Check sheet for the drawn part. Datum: minimum x, y, z corner. Units: mm. Coordinates: 2 decimals unless noted, no trailing zeros. Write each loop counter-clockwise with the first axis right and the second up, starting at its lowest first coordinate (ties: lowest second). Pieces come first, ordered by that corner, then holes. Notation, with made-up numbers: M 46.5,64.5 L 57.5,64.5 A28 cw 57.5,96.5 Z; hole C 55,-40 d4. An arc over 180 degrees is marked long. Answer as CSV lines item,"result". Start each with the question number.
Q1. Sectioned sample at B-B, the plane z = 61.13. Record the cut outline in (x, y), then the cut area to 3 significant figures.
Q2. Sectioned sample at D-D, the plane z = 93. Record the cut outline in (x, y).
Q3. Sectioned sample at A-A, the plane y = 1.45. Record the cut outline in (x, z), then the cut area to 3 significant figures.
Q4. Thickness scan on line 1 along Z through (x, y) = (40, 2.2); line 2 along Z through (x, y) = (38, 2.55); line 3 along X through (y, z) = (2.85, 58). Record the ranges inside material, lowest first. Write a range as from..to.
Q5. Sectioned sample at C-C, the plane x = 40. Record the cut outline in (y, z).
Q6. Depth check by flat-ended pin: pin 1 Ø0.9 at (x, y) = (75.5, 1.5) entering from -Z; pin 2 Ø0.9 at (y, z) = (1, 74.5) entering from +X; pin 3 Ø1.5 at (y, z) = (2, 31.5) entering from +X; pin 4 Ø1 at (x, y) = (27.5, 0.5) entering from -Z. Enter the tip coordinate at first touch or a pass-through.
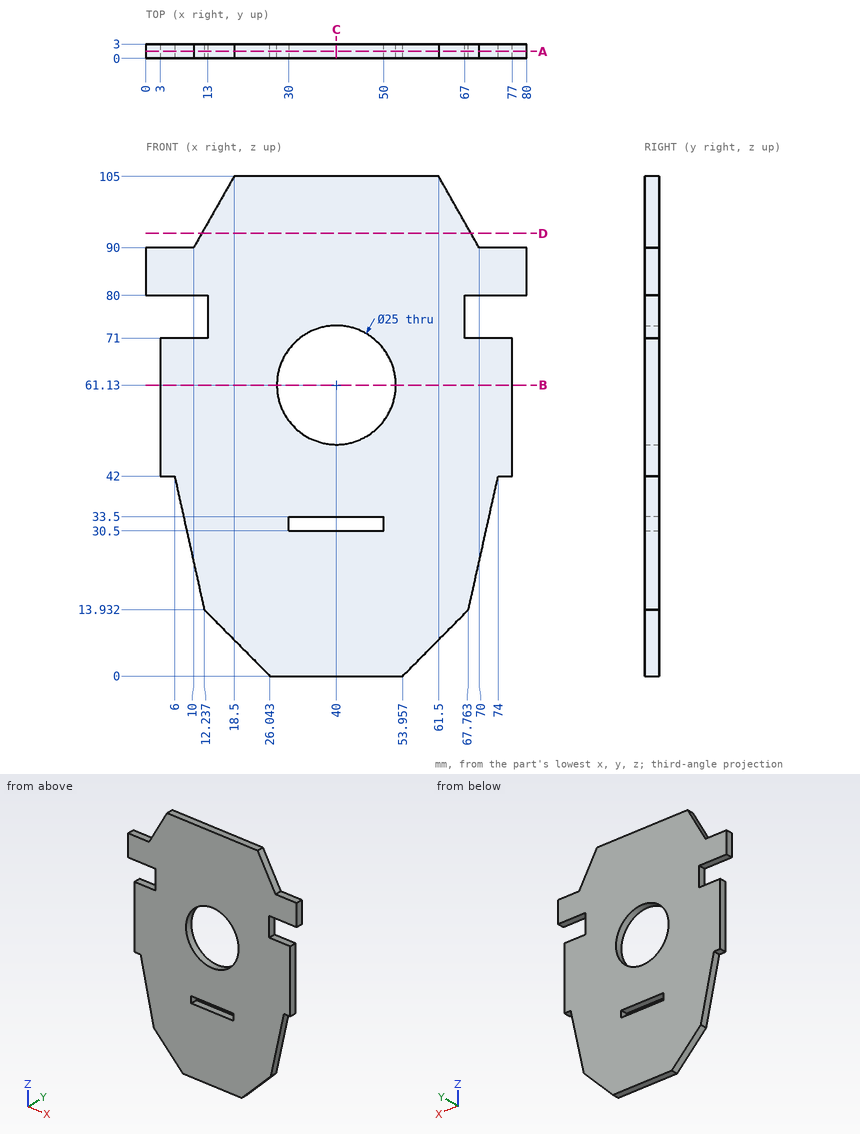
Output:
1,outline,"M 3,0 L 27.5,0 L 27.5,3 L 3,3 Z; M 52.5,0 L 77,0 L 77,3 L 52.5,3 Z"
1,area,"147 mm^2"
2,outline,"M 11.7,0 L 68.3,0 L 68.3,3 L 11.7,3 Z"
3,outline,"M 0,80 L 13,80 L 13,71 L 3,71 L 3,42 L 6,42 L 12.24,13.93 L 26.04,0 L 53.96,0 L 67.76,13.93 L 74,42 L 77,42 L 77,71 L 67,71 L 67,80 L 80,80 L 80,90 L 70,90 L 61.5,105 L 18.5,105 L 10,90 L 0,90 Z; hole C 40,61.13 d25; hole M 30,30.5 L 50,30.5 L 50,33.5 L 30,33.5 Z"
3,area,"5,970 mm^2"
4,line 1,"z = 0..30.5, 33.5..48.63, 73.63..105"
4,line 2,"z = 0..30.5, 33.5..48.79, 73.47..105"
4,line 3,"x = 3..27.9, 52.1..77"
5,outline,"M 0,0 L 3,0 L 3,30.5 L 0,30.5 Z; M 0,33.5 L 3,33.5 L 3,48.63 L 0,48.63 Z; M 0,73.63 L 3,73.63 L 3,105 L 0,105 Z"
6,pin 1,"stops at z = 42"
6,pin 2,"stops at x = 67"
6,pin 3,"stops at x = 71.83"
6,pin 4,"stops at z = 0"
